from build123d import *

# Parameters (mm, degrees)
SKETCH1_R           = 40
BOSS_EXTRUDE1_DEPTH = 15
FILLET1_R           = 5
SKETCH2_R           = 10
BOSS_EXTRUDE2_DEPTH = 25
SCALE1_SCALE        = 2
SKETCH3_W           = 67.082039325
SKETCH3_H           = 40
BOSS_EXTRUDE3_DEPTH = 50


with BuildPart() as part:
    # Sketch1 → Boss-Extrude1 (new body)
    with BuildSketch(Plane.XY):
        Circle(SKETCH1_R)
    extrude(amount=BOSS_EXTRUDE1_DEPTH)

    # Fillet1
    fillet1_edges = [part.edges().sort_by_distance(p)[0] for p in [
        (-40, 0, 15),
    ]]
    fillet(fillet1_edges, radius=FILLET1_R)

    # Sketch2 → Boss-Extrude2 (add)
    with BuildSketch(Plane.XY.offset(15)):
        Circle(SKETCH2_R)
    extrude(amount=BOSS_EXTRUDE2_DEPTH)


with BuildPart() as part_1:
    # Scale1: scaled about (0, 0, 9.31508132)
    add(part.part.scale(SCALE1_SCALE).moved(Location((0, 0, -9.31508132))))

    # Sketch3 → Boss-Extrude3 (add)
    with BuildSketch(Plane.XY.offset(70.68491868)):
        with Locations((33.541019663, 0)):
            Rectangle(SKETCH3_W, SKETCH3_H)
    extrude(amount=-BOSS_EXTRUDE3_DEPTH)


solid = part_1.part
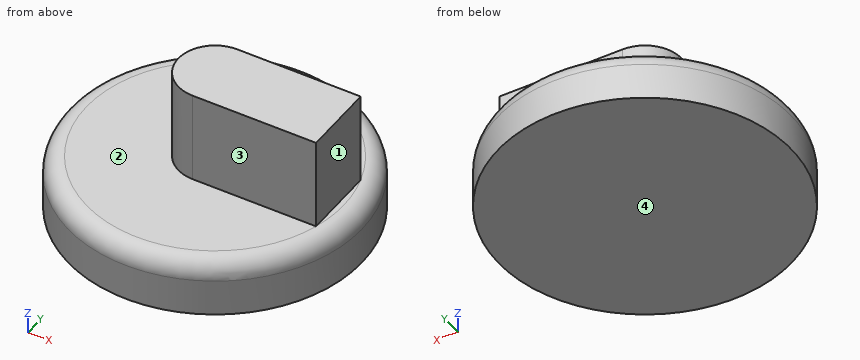
Source: CAD feature listing. Evaluate the final solid. Frame: model axes, mm. Face numbers are marked on the shaded views. A direction names the side the tool comes from. Coordinates: 2 decimals unless noted, no trailing zeros. Loops run counter-clockwise (first coordinate to the right, second up) from the corner with the lowest first, then second, coordinate; pieces in that order, holes last. Notation, with made-up numbers: (-35, -39.75) -> (-20, -39.75) arc R13 cw to (-20, -17.75) -> close; hole circle Ø5 at (-28, 21.5). An arc over 180 degrees is marked (long way). Answer in a Markdown table with one row per item. Add a question column.
Q1. Reachability of the marked faces 1, 2, 3 and 4 from +Z, -Z, +X, -X, +Y, -Y: full face, straight path, thin tool, end or side. Return the list, or none.
Q2. Section A-A on y = 0. Return the cut outline in (x, z), and give its area (3 significant figures).
Q3. Section B-B on z = 40. Return the cut outline in (x, y).
Q4. Ray query, line 1 along Y through (x, z) = (59, 63.5); line 2 along Z through (x, y) = (-39.5, -21.5); line 3 along X through (y, z) = (61.5, 13). Return the intervals inside material, ascending.
Q5. Contact query for flat-ended pins moving along their axis: pin 1 Ø20 at (y, z) = (-5.5, 37.5) entering from +X; pin 2 Ø1.5 at (x, y) = (69, 6) entering from +Z; pin 3 Ø6 at (y, z) = (-40, 14.5) entering from +X. Output: stop coordinate, or through.
Q6. Section C-C on z = 8.5. Return the cut outline in (x, y).
Computed values:
| question | item | result |
|---|---|---|
| 1 | face 1 | +Z, +X, +Y, -Y |
| 1 | face 2 | +Z, -X |
| 1 | face 3 | +Z, +X, -X, -Y |
| 1 | face 4 | -Z, +X, -X, +Y, -Y |
| 2 | outline | (-80, -9.32) -> (80, -9.32) -> (80, 10.68) arc R10 ccw to (70, 20.68) -> (67.08, 20.68) -> (67.08, 70.68) -> (-20, 70.68) -> (-20, 20.68) -> (-70, 20.68) arc R10 ccw to (-80, 10.68) -> close |
| 2 | area | 9,110 mm^2 |
| 3 | outline | (0, -20) -> (67.08, -20) -> (67.08, 20) -> (0, 20) arc R20 ccw to start |
| 4 | line 1 | y = -20 to 20 |
| 4 | line 2 | z = -9.32 to 20.68 |
| 4 | line 3 | x = -50.74 to 50.74 |
| 5 | pin 1 | stops at x = 67.08 |
| 5 | pin 2 | stops at z = 20.68 |
| 5 | pin 3 | stops at x = 70.41 |
| 6 | outline | circle Ø160 at (0, 0) |
